from build123d import *

# Parameters (mm, degrees)
F_8_32_TAPPED_HOLE1_D     = 3.4544
F_8_32_TAPPED_HOLE1_DEPTH = 10
F_8_32_TAPPED_HOLE1_TIP   = 1.037806461
CUT_EXTRUDE1_DEPTH        = 56


with BuildPart() as part:
    # Sketch1 → Revolve1 (revolve)
    with BuildSketch(Plane(origin=(0, 0, 0), x_dir=(1, 0, 0), z_dir=(0, 1, 0))):
        Polygon((4.6852, 0), (4.6852, 32), (7.227877139, 34.542677139), (8.3, 55), (8.55, 55), (8.8, 53), (8.8, 32), (8.8, 22), (9, 22), (9, 21), (8.8, 21), (8.8, 0), align=None)
    revolve(axis=Axis((0, 0, 0), (0, 0, -1)))

    # 8-32 Tapped Hole1
    with Locations(Plane(origin=(0, 8.8, -27), x_dir=(1, 0, 0), z_dir=(0, 1, 0))):
        with Locations((0, 0)):
            Hole(F_8_32_TAPPED_HOLE1_D / 2, depth=F_8_32_TAPPED_HOLE1_DEPTH)
            with Locations((0, 0, -(F_8_32_TAPPED_HOLE1_DEPTH + F_8_32_TAPPED_HOLE1_TIP / 2))):  # 118° drill point
                Cone(0, F_8_32_TAPPED_HOLE1_D / 2, F_8_32_TAPPED_HOLE1_TIP, mode=Mode.SUBTRACT)

    # Sketch3 → Cut-Extrude1 (cut, through all)
    with BuildSketch(Plane.XY):
        with BuildLine():
            Line((7.532191208, 4.926062891), (0, 0.577350269))
            Line((0, 0.577350269), (-7.532191208, 4.926062891))
            ThreePointArc((-7.532191208, 4.926062891), (0, -9), (7.532191208, 4.926062891))
        make_face()
    extrude(amount=-CUT_EXTRUDE1_DEPTH, mode=Mode.SUBTRACT)

    # Mirror1: part across plane


with BuildPart() as part_1:
    add(part.part)
    add(part.part.mirror(Plane(origin=(8.8, 0, 0), x_dir=(1, 0, 0), z_dir=(0, 0, 1))))


solid = part_1.part
The listing builds one solid part. Answer for the finished solid, in the listing's coordinates (mm). A direction names the side the tool comes from. Give positions to 0.01 mm unless a question says otherwise; leave off trailing zeros. Write each loop counter-clockwise with the first axis right and the second up, starting at its lowest first coordinate (ties: lowest second). Pieces come first, ordered by that corner, then holes. Notation, with made-up numbers: (-17, 61) -> (-4, 61) arc R21 ccw to (-4, 97) -> close; hole circle Ø8 at (-34, 42). An arc over 180 degrees is marked (long way). One line per question, with ' | ' between items. Start each with the question number.
1. Section D-D (z = 3) is taken. Determine the outline of the cut face in (x, y).
2. Find the intervals of material crossed by probe 1 along X at (y, z) = (6.45, -27); probe 2 along Z at (x, y) = (0, 6.3); probe 3 along Z at (x, y) = (0, 6.85), in increasing order.
3. Section A-A (x = 0) is taken. Determine the outline of the cut face in (y, z), plus the area to 3 significant figures.
4. Section B-B (z = 27) is taken. Determine the outline of the cut face in (x, y).
5. For a pull along X with two mould halves and no side action, classify faces 1 (the flat face through (-6.05, 4.07, -0.77)), 2 (the conical face through (-0.074, 5.409, -32.724)), 3 (the cylindrical face through (-0.1, 9, -21.5)) as pulls with the +X half, pulls with the -X half, needs draft (parallel to the pull), parting line crosses it, or undercut.
6. Section C-C (z = -46) is taken. Determine the outline of the cut face in (x, y), plus the area to 3 significant figures.
7. Given pin 1 Ø4 at (x, z) = (-0.5, 3.5) entering from -Y; pin 2 Ø8 at (x, z) = (4.5, -29.5) entering from -Y; pin 3 Ø3 at (y, z) = (7, 6) entering from +X; pin 4 Ø1 at (x, y) = (4.5, 4.5) entering from -Z, each flat-ended and moving along its own axis, determine where each tip first touches the part or whether it passes through.
8. For faces 4 (the cylindrical face through (1.726, 6.549, 27.076)), 5 (the conical face through (-0.074, 5.409, 32.724)), 6 (the cylindrical face through (-0.1, 8.8, -0.3)), 7 (the cylindrical face through (-0.1, 8.8, 37.7)), 8 (the cylindrical face through (-0.1, 8.8, -37.7)), determine the directions among +Z, -Z, +X, -X, +Y, -Y from which every point of the face is accessible in a straight line to the end or side of a thin tool.
Response values:
1) outline: (-7.36, 4.83) -> (-3.78, 2.76) arc R4.69 cw to (3.78, 2.76) -> (7.36, 4.83) arc R8.8 ccw to start
2) probe 1: -5.99 to -1.73, 1.73 to 5.99 | probe 2: -33.61 to -28.73, -25.27 to 25.27, 28.73 to 33.61 | probe 3: -34.16 to -28.73, -25.27 to 25.27, 28.73 to 34.16
3) outline: (4.69, -32) -> (7.23, -34.54) -> (8.3, -55) -> (8.55, -55) -> (8.8, -53) -> (8.8, -28.73) -> (4.69, -28.73) -> close; (4.69, -25.27) -> (8.8, -25.27) -> (8.8, -22) -> (9, -22) -> (9, -21) -> (8.8, -21) -> (8.8, 21) -> (9, 21) -> (9, 22) -> (8.8, 22) -> (8.8, 25.27) -> (4.69, 25.27) -> close; (4.69, 28.73) -> (8.8, 28.73) -> (8.8, 53) -> (8.55, 55) -> (8.3, 55) -> (7.23, 34.54) -> (4.69, 32) -> close | area: 292 mm2
4) outline: (-7.36, 4.83) -> (-3.78, 2.76) arc R4.69 cw to (-1.73, 4.36) -> (-1.73, 8.63) arc R8.8 ccw to start; (1.73, 4.36) arc R4.69 cw to (3.78, 2.76) -> (7.36, 4.83) arc R8.8 ccw to (1.73, 8.63) -> close
5) face 1: pulls with the -X half | face 2: undercut | face 3: parting line crosses it
6) outline: (-7.36, 4.83) -> (-6.52, 4.34) arc R7.83 cw to (6.52, 4.34) -> (7.36, 4.83) arc R8.8 ccw to start | area: 15.9 mm2
7) pin 1: y = 3.96 | pin 2: y = 2.76 | pin 3: x = 6.87 | pin 4: z = -34.18
8) face 4: +Y, -Y | face 5: +Z, -Y | face 6: +Y | face 7: +Z, +Y | face 8: -Z, +Y
